Verification items for the finished model (mm, model axes). A direction names the side the tool comes from. Round coordinates to 2 decimals unless told otherwise and drop trailing zeros. Loops run counter-clockwise (first coordinate to the right, second up) from the corner with the lowest first, then second, coordinate; pieces in that order, holes last. Notation, with made-up numbers: (21.25, 71) -> (73.25, 71) arc R11 ccw to (73.25, 90) -> close; hole circle Ø1 at (78.25, 19.5). An arc over 180 degrees is marked (long way). Use a Markdown table: item, result. Add a question column.
```python
from build123d import *

# Parameters (mm, degrees)
SKETCH1_R                = 15
BOSS_EXTRUDE1_DEPTH      = 190.5
SKETCH2_W                = 34
SKETCH2_H                = 34
BOSS_EXTRUDE2_DEPTH      = 17
SKETCH3_W                = 34
SKETCH3_H                = 34
BOSS_EXTRUDE3_DEPTH      = 15
CHAMFER2_SIZE            = 2.26
CHAMFER3_SIZE            = 0.707
SKETCH4_R                = 12.5
BOSS_EXTRUDE4_DEPTH      = 3
BOSS_EXTRUDE5_START      = 3
SKETCH5_R                = 12.5
BOSS_EXTRUDE5_DEPTH      = 3
SKETCH8_R                = 12
BOSS_EXTRUDE6_DEPTH      = 13
CHAMFER4_SIZE            = 0.5
BOSS_EXTRUDE7_START      = 13
SKETCH9_R                = 12
BOSS_EXTRUDE7_DEPTH      = 13
CHAMFER5_SIZE            = 0.5
CHAMFER6_SIZE            = 1
CHAMFER10_SIZE           = 1
SKETCH6_R                = 12.5
CUT_EXTRUDE1_DEPTH       = 152.5
SKETCH7_R                = 6
CUT_EXTRUDE2_DEPTH       = 208.89480513
CHAMFER7_SIZE            = 0.75
SKETCH10_R               = 3.5
SKETCH10_R_2             = 3.3
CUT_EXTRUDE3_DEPTH       = 2.5
SKETCH12_R               = 3.3
CUT_EXTRUDE4_DEPTH       = 0.5
CHAMFER8_SIZE            = 0.35
CUT_EXTRUDE5_DEPTH       = 2
SKETCH14_R               = 4
SKETCH14_R_2             = 3.5
CUT_EXTRUDE6_DEPTH       = 0.5
CHAMFER9_SIZE            = 0.5
CHAMFER8_OF_MIRROR1_SIZE = 0.35
CHAMFER9_OF_MIRROR1_SIZE = 0.5
SKETCH19_R               = 1.5
CUT_EXTRUDE8_DEPTH       = 6
CHAMFER11_SIZE           = 0.5
G1_8_TAPPED_HOLE1_D      = 8.566
G1_8_TAPPED_HOLE1_DEPTH  = 25
G1_8_TAPPED_HOLE1_TIP    = 2.573486031


with BuildPart() as part:
    # Sketch1 → Boss-Extrude1 (new, symmetric)
    with BuildSketch(Plane.XY):
        Circle(SKETCH1_R)
    extrude(amount=BOSS_EXTRUDE1_DEPTH, both=True)

    # Sketch2 → Boss-Extrude2 (add)
    with BuildSketch(Plane.XY.offset(190.5)):
        Rectangle(SKETCH2_W, SKETCH2_H)
    extrude(amount=-BOSS_EXTRUDE2_DEPTH)

    # Sketch3 → Boss-Extrude3 (add)
    with BuildSketch(Plane(origin=(0, 0, -190.5), x_dir=(-1, 0, 0), z_dir=(0, 0, -1))):
        Rectangle(SKETCH3_W, SKETCH3_H)
    extrude(amount=-BOSS_EXTRUDE3_DEPTH)

    # Chamfer2
    chamfer2_edges = [part.edges().sort_by_distance(p)[0] for p in [
        (-17, 17, -183),
        (-17, -17, -183),
        (17, -17, -183),
        (17, 17, -183),
        (17, 17, 182),
        (17, -17, 182),
        (-17, -17, 182),
        (-17, 17, 182),
    ]]
    chamfer(chamfer2_edges, length=CHAMFER2_SIZE)

    # Chamfer3
    chamfer3_edges = [part.edges().sort_by_distance(p)[0] for p in [
        (-17, 0, -190.5),
        (17, 0, -190.5),
        (-15.87, 15.87, -190.5),
        (15.87, 15.87, -190.5),
        (15.87, -15.87, -190.5),
        (-15.87, -15.87, -190.5),
        (-17, 0, -175.5),
        (17, 0, -175.5),
        (-15.87, 15.87, -175.5),
        (15.87, 15.87, -175.5),
        (15.87, -15.87, -175.5),
        (-15.87, -15.87, -175.5),
        (-17, 0, 190.5),
        (-17, 0, 173.5),
        (17, 0, 190.5),
        (15.87, 15.87, 190.5),
        (-15.87, 15.87, 190.5),
        (15.87, -15.87, 190.5),
        (-15.87, -15.87, 190.5),
        (17, 0, 173.5),
        (15.87, 15.87, 173.5),
        (-15.87, 15.87, 173.5),
        (15.87, -15.87, 173.5),
        (-15.87, -15.87, 173.5),
    ]]
    chamfer(chamfer3_edges, length=CHAMFER3_SIZE)

    # Sketch4 → Boss-Extrude4 (add)
    with BuildSketch(Plane(origin=(0, 0, -190.5), x_dir=(-1, 0, 0), z_dir=(0, 0, -1))):
        with Locations(Location((0, 0, 0), (0, 0, 180))):
            Circle(SKETCH4_R)
    extrude(amount=BOSS_EXTRUDE4_DEPTH)

    # Sketch5 → Boss-Extrude5 (add)
    with BuildSketch(Plane.XY.offset(190.5).offset(BOSS_EXTRUDE5_START)):
        Circle(SKETCH5_R)
    extrude(amount=-BOSS_EXTRUDE5_DEPTH)

    # Sketch8 → Boss-Extrude6 (add)
    with BuildSketch(Plane.XY.offset(193.5)):
        with Locations(Location((0, 0, 0), (0, 0, 180))):
            Circle(SKETCH8_R)
    extrude(amount=BOSS_EXTRUDE6_DEPTH)

    # Chamfer4
    chamfer4_edges = [part.edges().sort_by_distance(p)[0] for p in [
        (12, 0, 193.5),
    ]]
    chamfer(chamfer4_edges, length=CHAMFER4_SIZE - 0.0001)  # a hair under: the kernel refuses the full size

    # Sketch9 → Boss-Extrude7 (add)
    with BuildSketch(Plane(origin=(0, 0, -193.5), x_dir=(-1, 0, 0), z_dir=(0, 0, -1)).offset(BOSS_EXTRUDE7_START)):
        Circle(SKETCH9_R)
    extrude(amount=-BOSS_EXTRUDE7_DEPTH)

    # Chamfer5
    chamfer5_edges = [part.edges().sort_by_distance(p)[0] for p in [
        (12, 0, -193.5),
    ]]
    chamfer(chamfer5_edges, length=CHAMFER5_SIZE - 0.0001)  # a hair under: the kernel refuses the full size

    # Chamfer6
    chamfer6_edges = [part.edges().sort_by_distance(p)[0] for p in [
        (12, 0, 206.5),
    ]]
    chamfer(chamfer6_edges, length=CHAMFER6_SIZE)

    # Chamfer10
    chamfer10_edges = [part.edges().sort_by_distance(p)[0] for p in [
        (12, 0, -206.5),
    ]]
    chamfer(chamfer10_edges, length=CHAMFER10_SIZE)

    # Sketch6 → Cut-Extrude1 (cut, symmetric)
    with BuildSketch(Plane.XY):
        Circle(SKETCH6_R)
    extrude(amount=CUT_EXTRUDE1_DEPTH, both=True, mode=Mode.SUBTRACT)

    # Sketch7 → Cut-Extrude2 (cut, through all)
    with BuildSketch(Plane.XY):
        Circle(SKETCH7_R)
    extrude(amount=CUT_EXTRUDE2_DEPTH, mode=Mode.SUBTRACT)

    # Chamfer7
    chamfer7_edges = [part.edges().sort_by_distance(p)[0] for p in [
        (-6, 0, 206.5),
    ]]
    chamfer(chamfer7_edges, length=CHAMFER7_SIZE)

    # Sketch10 → Cut-Extrude3 (cut)
    with BuildSketch(Plane(origin=(0, 17, 0), x_dir=(1, 0, 0), z_dir=(0, 1, 0))):
        with Locations(Location((-9.5, -178.5, 0), (0, 0, 270))):
            Circle(SKETCH10_R)
        with Locations(Location((-9.5, -178.5, 0), (0, 0, 270))):
            Circle(SKETCH10_R_2, mode=Mode.SUBTRACT)
    cut_extrude3 = extrude(amount=-CUT_EXTRUDE3_DEPTH, mode=Mode.SUBTRACT)

    # Sketch12 → Cut-Extrude4 (cut)
    with BuildSketch(Plane(origin=(0, 17, 0), x_dir=(1, 0, 0), z_dir=(0, 1, 0))):
        with Locations(Location((-9.5, -178.5, 0), (0, 0, 270))):
            Circle(SKETCH12_R)
    cut_extrude4 = extrude(amount=-CUT_EXTRUDE4_DEPTH, mode=Mode.SUBTRACT)

    # Chamfer8
    chamfer8_edges = [part.edges().sort_by_distance(p)[0] for p in [
        (-9.5, 16.5, 175.2),
    ]]
    chamfer(chamfer8_edges, length=CHAMFER8_SIZE)

    # Sketch13 → Cut-Extrude5 (cut)
    with BuildSketch(Plane(origin=(0, 16.5, 0), x_dir=(1, 0, 0), z_dir=(0, 1, 0))):
        Polygon((-7.825684219, -178.5), (-8.66284211, -177.05), (-10.33715789, -177.05), (-11.174315781, -178.5), (-10.33715789, -179.95), (-8.66284211, -179.95), align=None)
    cut_extrude5 = extrude(amount=-CUT_EXTRUDE5_DEPTH, mode=Mode.SUBTRACT)

    # Sketch14 → Cut-Extrude6 (cut)
    with BuildSketch(Plane(origin=(0, 17, 0), x_dir=(1, 0, 0), z_dir=(0, 1, 0))):
        with Locations(Location((-9.5, -178.5, 0), (0, 0, 270))):
            Circle(SKETCH14_R)
        with Locations(Location((-9.5, -178.5, 0), (0, 0, 270))):
            Circle(SKETCH14_R_2, mode=Mode.SUBTRACT)
    cut_extrude6 = extrude(amount=-CUT_EXTRUDE6_DEPTH, mode=Mode.SUBTRACT)

    # Chamfer9
    chamfer9_edges = [part.edges().sort_by_distance(p)[0] for p in [
        (-9.5, 16.5, 174.5),
    ]]
    chamfer(chamfer9_edges, length=CHAMFER9_SIZE - 0.0001)  # a hair under: the kernel refuses the full size

    # Mirror1: Cut-Extrude3, Cut-Extrude4, Cut-Extrude5, Cut-Extrude6 across plane
    add(cut_extrude3.mirror(Plane.XY.offset(-1)), mode=Mode.SUBTRACT)
    add(cut_extrude4.mirror(Plane.XY.offset(-1)), mode=Mode.SUBTRACT)
    add(cut_extrude5.mirror(Plane.XY.offset(-1)), mode=Mode.SUBTRACT)
    add(cut_extrude6.mirror(Plane.XY.offset(-1)), mode=Mode.SUBTRACT)

    # Chamfer8 of Mirror1
    chamfer8_of_mirror1_edges = [part.edges().sort_by_distance(p)[0] for p in [
        (-9.5, 16.5, -177.2),
    ]]
    chamfer(chamfer8_of_mirror1_edges, length=CHAMFER8_OF_MIRROR1_SIZE)

    # Chamfer9 of Mirror1
    chamfer9_of_mirror1_edges = [part.edges().sort_by_distance(p)[0] for p in [
        (-9.5, 16.5, -176.5),
    ]]
    chamfer(chamfer9_of_mirror1_edges, length=CHAMFER9_OF_MIRROR1_SIZE - 0.0001)  # a hair under: the kernel refuses the full size

    # Sketch19 → Cut-Extrude8 (cut)
    with BuildSketch(Plane(origin=(17, 0, 0), x_dir=(0, 0, -1), z_dir=(1, 0, 0))):
        with Locations((-178.5, 0)):
            Circle(SKETCH19_R)
    cut_extrude8 = extrude(amount=-CUT_EXTRUDE8_DEPTH, mode=Mode.SUBTRACT)

    # Mirror3: Cut-Extrude8 across plane
    add(cut_extrude8.mirror(Plane.XY.offset(-1)), mode=Mode.SUBTRACT)

    # Chamfer11
    chamfer11_edges = [part.edges().sort_by_distance(p)[0] for p in [
        (17, 0, 180),
        (17, 0, -182),
    ]]
    chamfer(chamfer11_edges, length=CHAMFER11_SIZE)

    # G1/8 Tapped Hole1
    with Locations(Plane(origin=(0, 17, 0), x_dir=(-1, 0, 0), z_dir=(0, 1, 0))):
        with Locations((-6, 180.5), (-6, -182.5)):
            Hole(G1_8_TAPPED_HOLE1_D / 2, depth=G1_8_TAPPED_HOLE1_DEPTH)
            with Locations((0, 0, -(G1_8_TAPPED_HOLE1_DEPTH + G1_8_TAPPED_HOLE1_TIP / 2))):  # 118° drill point
                Cone(0, G1_8_TAPPED_HOLE1_D / 2, G1_8_TAPPED_HOLE1_TIP, mode=Mode.SUBTRACT)


solid = part.part
```
1) Thickness scan on line 1 (Z direction, x = 6, y = 10.5); line 2 (Y direction, x = 14.8, z = 178.5); line 3 (Y direction, x = 0.5, z = -63). Record the ranges inside material, lowest first.
2) Sectioned sample at A-A on z = -79. Enter the section's corners in (x, y), then the cut area to 3 significant figures.
3) Access from +Z, -Z, +X, -X, +Y, -Y to the whole of each face (thin tool, end or side, straight path). Record for faces 1 (the face through (11, 8, -190.5)), 2 (the face through (0, -17, -183)), 3 (the face through (-14.985, 0.66, 1.443)), 4 (the face through (-11.446, -3.604, 199.669)), 5 (the face through (10.085, 4.325, 181.786)).
4) Release check for a two-part mould opening along X. For faces 6 (the face through (17, 0, 182)), 7 (the face through (-9.4, 15.3, 175.2)), 8 (the face through (0, 0, -206.5)) record: released by +X, released by -X, zero draft, split by the parting line, or undercut.
5) Go/stop test with flat-tipped pins: pin 1 (3 mm diameter, centred on x = -11, y = 6, fed in from +Z); pin 2 (0.9 mm diameter, centred on y = 0.5, z = 178.5, fed in from +X); pin 3 (1 mm diameter, centred on x = -11.5, z = -154.5, fed in from +Y). Record where each tip stops, or that it passes through.
6) Sectioned sample at B-B on z = -157. Enter the section's corners in (x, y), then the cut area to 3 significant figures.
Geometry results:
| question | item | result |
|---|---|---|
| 1 | line 1 | -193.91 to -186.78, -178.22 to -152.5, 152.5 to 176.22, 184.78 to 193.91 |
| 1 | line 2 | -16.94 to -1.5, 1.5 to 16.94 |
| 1 | line 3 | -14.99 to -12.49, 12.49 to 14.99 |
| 2 | outline | circle Ø30 at (0, 0); hole circle Ø25 at (0, 0) |
| 2 | area | 216 mm^2 |
| 3 | face 1 | -Z |
| 3 | face 2 | +Z, -Z, +X, -X, -Y |
| 3 | face 3 | none |
| 3 | face 4 | +Z |
| 3 | face 5 | +Y |
| 4 | face 6 | released by +X |
| 4 | face 7 | undercut |
| 4 | face 8 | zero draft |
| 5 | pin 1 | z = 206.47 |
| 5 | pin 2 | x = 11 |
| 5 | pin 3 | y = 10.2 |
| 6 | outline | circle Ø30 at (0, 0) |
| 6 | area | 707 mm^2 |
